Can you work these out from the drawing? Everything is in mm from the part's minimum corner. Coordinates: 2 decimals unless noted, no trailing zeros. Loops run counter-clockwise (first coordinate to the right, second up) from the corner with the lowest first, then second, coordinate; pieces in that order, holes last. Notation, with made-up numbers: M -20,8.25 L 17,8.25 A26 ccw 17,38.25 Z; hole C 77.5,-36 d10. An arc over 180 degrees is marked long. Write each question's results on one line, items separated by ' | '.
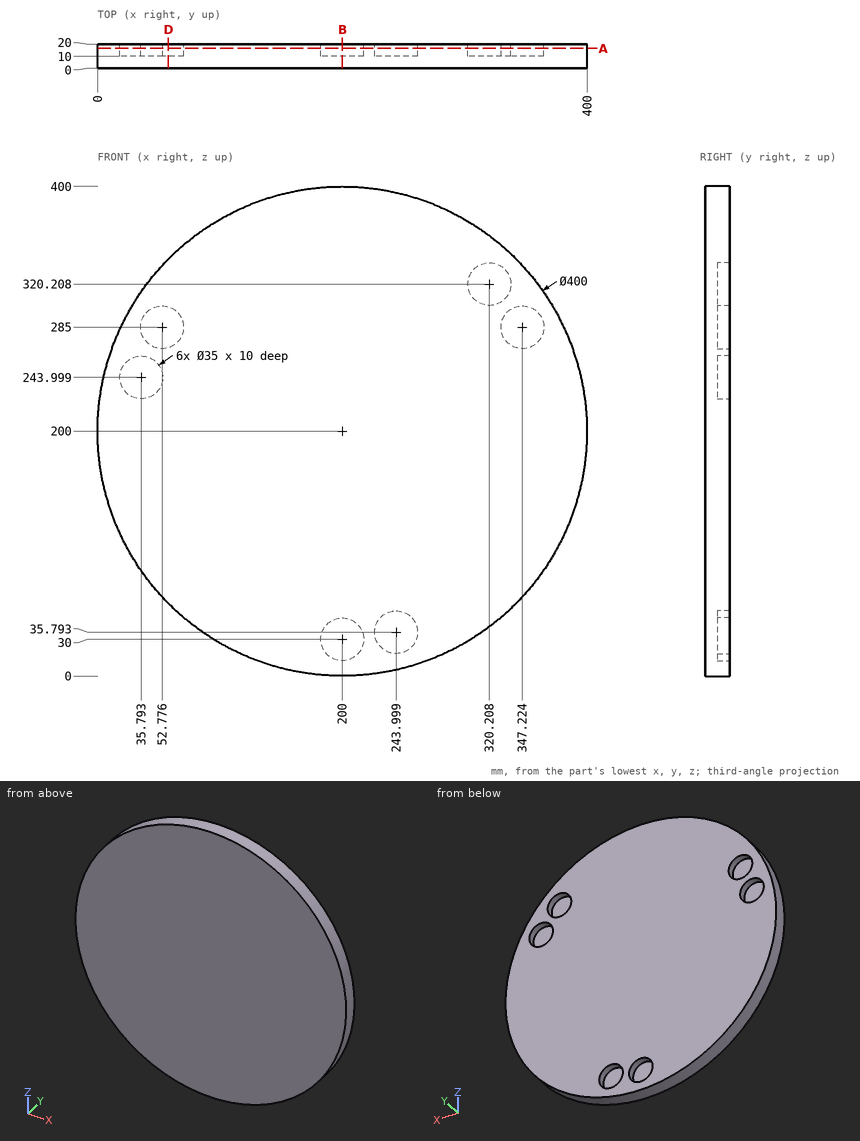
(1) Will these pins go through, and if not, where does the flat tip stop? P1, Ø21, axis at x = 35.79, z = 244, coming from the +Y side; P2, Ø10, axis at y = 12.5, z = 282.5, coming from the +X side; P3, Ø2, axis at y = 17.5, z = 98.5, coming from the +X side (1 decimal).
Reported:
P1: stops at y = 10 | P2: stops at x = 384.37 | P3: stops at x = 372.9
(2) Imagine slicing it at A-A, the plane y = 16.5. List the corners of the cut face in (x, z) for me (1 decimal), and give its area (3 significant figures).
Reported:
outline: C 200,200 d400; hole C 35.8,244 d35; hole C 52.8,285 d35; hole C 200,30 d35; hole C 244,35.8 d35; hole C 320.2,320.2 d35; hole C 347.2,285 d35 | area: 120,000 mm2
(3) Imagine slicing it at B-B, the plane x = 200. List the corners of the cut face in (y, z) for me.
Reported:
outline: M 0,0 L 20,0 L 20,12.5 L 10,12.5 L 10,47.5 L 20,47.5 L 20,400 L 0,400 Z
(4) Please list where these lines run through material, in increasing order: probe 1 along X at (y, z) = (15, 285) (1 decimal); probe 2 along X at (y, z) = (12.5, 30) (1 decimal); probe 3 along Z at (x, y) = (30, 19) (1 decimal). Write a range as from..to.
Reported:
probe 1: x = 19..35.3, 70.3..329.7, 364.7..381 | probe 2: x = 94.6..182.5, 217.5..227.5, 260.5..305.4 | probe 3: z = 94.6..227.5, 260.5..305.4
(5) Imagine slicing it at D-D, the plane x = 58. List the corners of the cut face in (y, z) for me.
Reported:
outline: M 0,59.16 L 20,59.16 L 20,268.3 L 10,268.3 L 10,301.7 L 20,301.7 L 20,340.84 L 0,340.84 Z
